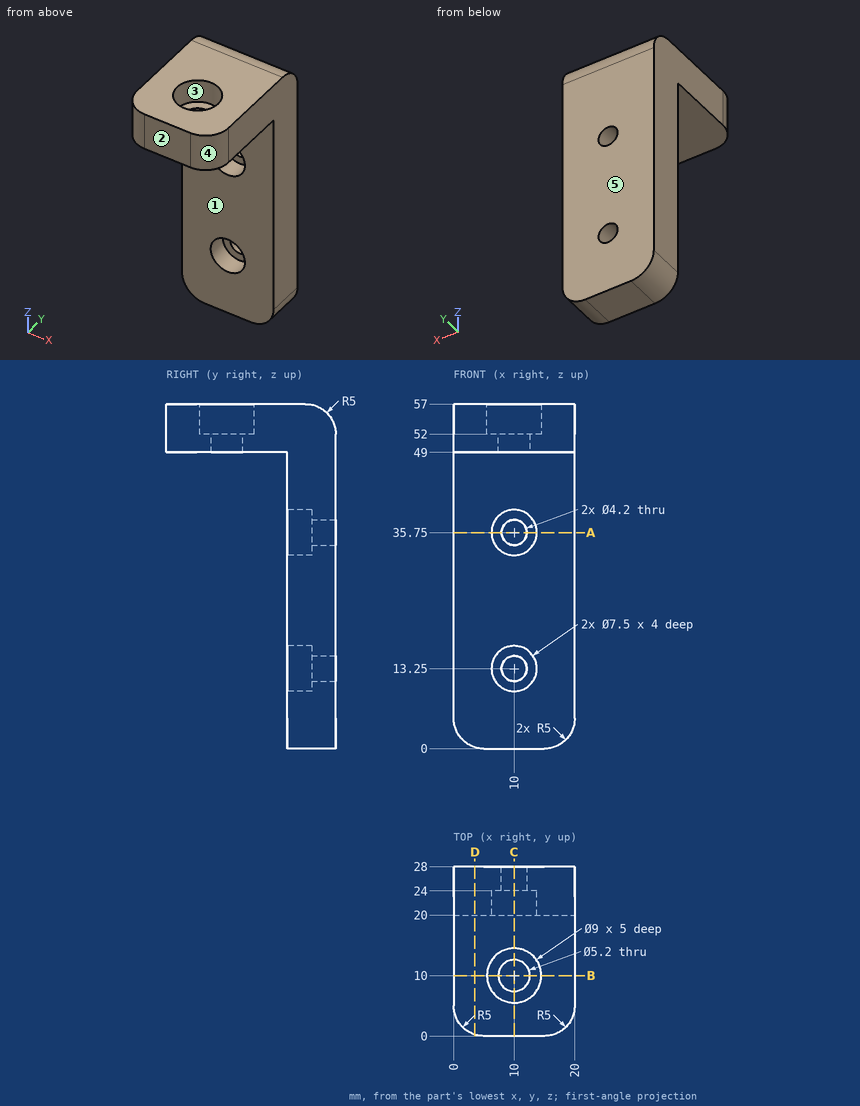
Geometry check sheet. Reference: drawing and pictorial views, mm from the part's lowest x, y, z. A direction names the side the tool comes from. Give positions to 0.01 mm unless a question says otherwise; leave off trailing zeros. Write each loop counter-clockwise with the first axis right and the second up, starting at its lowest first coordinate (ties: lowest second). Pieces come first, ordered by that corner, then holes. Notation, with made-up numbers: (33.25, 74.5) - (84.25, 74.5) arc R15 cw to (84.25, 89.5) - close; hole circle Ø7 at (-5.5, 7.25). An arc over 180 degrees is marked (long way). Put each result on its own line as item: value.
Q1. Scan lines: probe 1 along Z at (x, y) = (10, 21.2); probe 2 along X at (y, z) = (25.65, 13.25); probe 3 along Z at (x, y) = (19.25, 2.5). Record each from-to range of solid material in increasing order. Write a range as from..to.
Result:
probe 1: 0..9.5, 17..32, 39.5..57
probe 2: 0..7.9, 12.1..20
probe 3: 49..57
Q2. Section check A-A on z = 35.75. Record the cut outline in (x, y).
Result:
outline: (0, 20) - (6.25, 20) - (6.25, 24) - (7.9, 24) - (7.9, 28) - (0, 28) - close; (12.1, 24) - (13.75, 24) - (13.75, 20) - (20, 20) - (20, 28) - (12.1, 28) - close
Q3. Depth check by flat-ended pin: P1, Ø1.5, axis at x = 5, z = 36, coming from the -Y side; P2, Ø7, axis at x = 10, y = 10, coming from the -Z side; P3, Ø7, axis at x = 10.5, y = 10.5, coming from the +Z side. Enter the tip coordinate at first touch or a pass-through.
Result:
P1: y = 20
P2: z = 49
P3: z = 52
Q4. Mould release check, pull along X, two halves, no side actions. Record for the marked faces 3, 4 and 5: released by +X, released by -X, zero draft, split by the parting line, or undercut.
Result:
face 3: undercut
face 4: released by +X
face 5: zero draft
Q5. Section check D-D on x = 3.5. Record the cut outline in (y, z).
Result:
outline: (0.23, 49) - (20, 49) - (20, 0.23) - (28, 0.23) - (28, 52) arc R5 ccw to (23, 57) - (0.23, 57) - close
Q6. Set-up check for the marked faces 1 and 2: record each of +Z, -Z, +X, -X, +Y, -Y from which the full face is reachable in a straight line by a thin tool's end or side.
Result:
face 1: -Z, +X, -X, -Y
face 2: +Z, -Z, +X, -X, -Y
Q7. Section check C-C on x = 10. Count the separate pieces of the cut face and the enclosed holes in it, and give its area (3 significant figures).
Result:
separate pieces: 4
enclosed holes: 0
area: 456 mm2
Q8. Section check B-B on y = 10. Record the cut outline in (x, z), and give its area (3 significant figures).
Result:
outline: (0, 49) - (7.4, 49) - (7.4, 52) - (5.5, 52) - (5.5, 57) - (0, 57) - close; (12.6, 49) - (20, 49) - (20, 57) - (14.5, 57) - (14.5, 52) - (12.6, 52) - close
area: 99.4 mm2
